from build123d import *

# Parameters (mm, degrees)
SKETCH1_W           = 42
SKETCH1_H           = 42
SKETCH1_W_2         = 38
SKETCH1_H_2         = 38
BOSS_EXTRUDE1_DEPTH = 250
BOSS_EXTRUDE2_DEPTH = 21
CUT_EXTRUDE1_REACH  = 356.177
SKETCH3_R           = 6.5
CUT_EXTRUDE2_REACH  = 356.177
SKETCH4_R           = 3
SKETCH5_W           = 175
SKETCH5_H           = 38
CUT_EXTRUDE3_DEPTH  = 10
SKETCH6_R           = 2
CUT_EXTRUDE4_DEPTH  = 354.396378023


with BuildPart() as part:
    # Sketch1 → Boss-Extrude1 (new body)
    with BuildSketch(Plane.XY):
        Rectangle(SKETCH1_W, SKETCH1_H)
        Rectangle(SKETCH1_W_2, SKETCH1_H_2, mode=Mode.SUBTRACT)
    extrude(amount=-BOSS_EXTRUDE1_DEPTH)

    # Sketch2 → Boss-Extrude2 (add, symmetric)
    with BuildSketch(Plane(origin=(0, 0, 0), x_dir=(1, 0, 0), z_dir=(0, 1, 0))):
        Polygon((-25, 250), (-25, 350), (-23, 350), (-23, 252), (23, 252), (23, 350), (25, 350), (25, 250), align=None)
    extrude(amount=BOSS_EXTRUDE2_DEPTH, both=True)

    # Sketch3 → Cut-Extrude1 (cut, up to next)
    with BuildSketch(Plane.ZY.offset(25), mode=Mode.PRIVATE) as cut_extrude1_sk1:
        with Locations((-25, 0)):
            Circle(SKETCH3_R)
    cut_extrude1_tool1 = extrude(cut_extrude1_sk1.sketch, amount=-CUT_EXTRUDE1_REACH, mode=Mode.PRIVATE) & part.part
    # Sketch3 → Cut-Extrude1 (cut, up to next)
    with BuildSketch(Plane.ZY.offset(25), mode=Mode.PRIVATE) as cut_extrude1_sk2:
        with Locations((-325, 0)):
            Circle(SKETCH3_R)
    cut_extrude1_tool2 = extrude(cut_extrude1_sk2.sketch, amount=-CUT_EXTRUDE1_REACH, mode=Mode.PRIVATE) & part.part
    add(cut_extrude1_tool1.solids().sort_by_distance((-25, 0, -25))[0], mode=Mode.SUBTRACT)
    add(cut_extrude1_tool2.solids().sort_by_distance((-25, 0, -325))[0], mode=Mode.SUBTRACT)

    # Sketch4 → Cut-Extrude2 (cut, up to next)
    with BuildSketch(Plane(origin=(25, 0, 0), x_dir=(0, 0, -1), z_dir=(1, 0, 0)), mode=Mode.PRIVATE) as cut_extrude2_sk1:
        with Locations((325, 0)):
            Circle(SKETCH4_R)
    cut_extrude2_tool1 = extrude(cut_extrude2_sk1.sketch, amount=-CUT_EXTRUDE2_REACH, mode=Mode.PRIVATE) & part.part
    # Sketch4 → Cut-Extrude2 (cut, up to next)
    with BuildSketch(Plane(origin=(25, 0, 0), x_dir=(0, 0, -1), z_dir=(1, 0, 0)), mode=Mode.PRIVATE) as cut_extrude2_sk2:
        with Locations((25, 0)):
            Circle(SKETCH4_R)
    cut_extrude2_tool2 = extrude(cut_extrude2_sk2.sketch, amount=-CUT_EXTRUDE2_REACH, mode=Mode.PRIVATE) & part.part
    add(cut_extrude2_tool1.solids().sort_by_distance((25, 0, -325))[0], mode=Mode.SUBTRACT)
    add(cut_extrude2_tool2.solids().sort_by_distance((25, 0, -25))[0], mode=Mode.SUBTRACT)

    # Sketch5 → Cut-Extrude3 (cut)
    with BuildSketch(Plane(origin=(21, 0, 0), x_dir=(0, 0, -1), z_dir=(1, 0, 0))):
        with Locations((142.5, 0)):
            Rectangle(SKETCH5_W, SKETCH5_H)
    extrude(amount=-CUT_EXTRUDE3_DEPTH, mode=Mode.SUBTRACT)

    # Sketch6 → Cut-Extrude4 (cut, through all)
    with BuildSketch(Plane(origin=(0, 21, 0), x_dir=(1, 0, 0), z_dir=(0, 1, 0))):
        with Locations(Location((2, 25, 0), (0, 0, 270))):
            Circle(SKETCH6_R)
    extrude(amount=-CUT_EXTRUDE4_DEPTH, mode=Mode.SUBTRACT)


solid = part.part
Input: part model. Units: mm. Frame: model coordinates. A direction names the side the tool comes from. Coordinates: 2 decimals unless noted, no trailing zeros. Order: outer loops, then holes, each group sorted by start corner. A loop starts at its lowest first (then second) coordinate and runs counter-clockwise, first axis right, second up. Notation, with made-up numbers: M 5.25,39 L 55.25,39 A18 ccw 55.25,55 Z; hole C 66.5,5 d5. An arc over 180 degrees is marked long. Answer in a Markdown table with one row per item.
(1) Contact query for flat-ended pins moving along their axis: pin 1 Ø12 at (x, y) = (10.5, 2.5) entering from -Z; pin 2 Ø19 at (y, z) = (-4, -118) entering from +X; pin 3 Ø4 at (x, y) = (11.5, -12.5) entering from +Z. Output: stop coordinate, or through.
Numbers:
| item | result |
|---|---|
| pin 1 | stops at z = -252 |
| pin 2 | stops at x = -19 |
| pin 3 | stops at z = -250 |
(2) Section query C-C, the plane z = -141.5. Output: boundary loops of the cut face in (x, y), plus the area to 3 significant figures.
Numbers:
| item | result |
|---|---|
| outline | M -21,-21 L 21,-21 L 21,-19 L -19,-19 L -19,19 L 21,19 L 21,21 L -21,21 Z |
| area | 244 mm^2 |
(3) Section query B-B, the plane z = -325. Output: boundary loops of the cut face in (x, y), plus the area to 3 significant figures.
Numbers:
| item | result |
|---|---|
| outline | M -25,-21 L -23,-21 L -23,-6.5 L -25,-6.5 Z; M -25,6.5 L -23,6.5 L -23,21 L -25,21 Z; M 23,-21 L 25,-21 L 25,-3 L 23,-3 Z; M 23,3 L 25,3 L 25,21 L 23,21 Z |
| area | 130 mm^2 |
(4) Section query D-D, the plane x = -11. Output: boundary loops of the cut face in (y, z), plus the area to 3 significant figures.
Numbers:
| item | result |
|---|---|
| outline | M -21,-252 L 21,-252 L 21,0 L 19,0 L 19,-250 L -19,-250 L -19,0 L -21,0 Z |
| area | 1,080 mm^2 |
(5) Section query A-A, the plane y = -14.5. Output: boundary loops of the cut face in (x, z).
Numbers:
| item | result |
|---|---|
| outline | M -25,-350 L -23,-350 L -23,-252 L 23,-252 L 23,-350 L 25,-350 L 25,-250 L 21,-250 L 21,-230 L 19,-230 L 19,-250 L -19,-250 L -19,0 L -21,0 L -21,-250 L -25,-250 Z; M 19,-55 L 21,-55 L 21,0 L 19,0 Z |
(6) Access query for faces 1 (the cylindrical face through (-24.01, 1.95, -318.8)), 2 (the flat face through (-21, 0, -123)), 3 (the flat face through (0, 0, -252)), 4 (the flat face through (-19, 0, -123)). Directions: +Z, -Z, +X, -X, +Y, -Y. A direction counts if a zero-diameter tool reaches every point of the face in a straight line with its end or side. Return the directions, or none.
Numbers:
| item | result |
|---|---|
| face 1 | -X |
| face 2 | +Z, -X, +Y, -Y |
| face 3 | -Z, +Y, -Y |
| face 4 | +Z |
(7) Draft query along X for faces 5 (the flat face through (0, 0, -250)), 6 (the flat face through (-2, -20, 0)), 7 (the flat face through (21, 20, -87)). Return one class per face: pulls with the +X half, pulls with the -X half, needs draft (parallel to the pull), parting line crosses it, or undercut.
Numbers:
| item | result |
|---|---|
| face 5 | undercut |
| face 6 | needs draft |
| face 7 | pulls with the +X half |
(8) Material intervals for line 1 (Y direction, x = 20.3, z = -25); line 2 (X direction, y = 18, z = -293); line 3 (Y direction, x = -4, z = -145.5), sorted ascending. Write a range as [from, to].
Numbers:
| item | result |
|---|---|
| line 1 | y = [-21, -3], [3, 21] |
| line 2 | x = [-25, -23], [23, 25] |
| line 3 | y = [-21, -19], [19, 21] |
